```python
from build123d import *

# Parameters (mm, degrees)
BOSS_EXTRUDE1_DEPTH     = 60.96
SKETCH4_R               = 12.065
CUT_EXTRUDE3_DEPTH      = 3.81
CUT_EXTRUDE4_DEPTH      = 1
CUT_EXTRUDE4_DEPTH_BACK = 102.872142857
SKETCH7_R               = 3.81
BOSS_EXTRUDE3_DEPTH     = 3.81
CUT_EXTRUDE7_DEPTH      = 3.81
SKETCH11_R              = 12.065
CUT_EXTRUDE8_DEPTH      = 114.3


with BuildPart() as part:
    # Sketch1 → Boss-Extrude1 (new body)
    with BuildSketch(Plane.XY):
        with BuildLine():
            Line((40.776071429, -15.784285714), (40.776071429, 14.695714286))
            ThreePointArc((40.776071429, 14.695714286), (38.819326582, 21.468636013), (33.552060607, 26.154490072))
            Line((33.552060607, 26.154490072), (-40.503928571, 26.154490072))
            ThreePointArc((-40.503928571, 26.154490072), (-42.006230477, 20.457549787), (-40.776071429, 14.695714286))
            Line((-40.776071429, 14.695714286), (-40.776071429, -15.784285714))
            Line((-40.776071429, -15.784285714), (-50.936071429, -15.784285714))
            Line((-50.936071429, -15.784285714), (-50.936071429, 39.587714286))
            ThreePointArc((-50.936071429, 39.587714286), (-48.041649354, 41.212124157), (-44.960126074, 42.445250611))
            ThreePointArc((-44.960126074, 42.445250611), (-42.948064089, 46.137564922), (-42.251938956, 50.284490072))
            Line((-42.251938956, 50.284490072), (-29.309810678, 50.284490072))
            Line((-29.309810678, 50.284490072), (29.309810678, 50.284490072))
            Line((29.309810678, 50.284490072), (42.251938956, 50.284490072))
            Line((42.251938956, 50.284490072), (42.251938956, 48.042823233))
            ThreePointArc((42.251938956, 48.042823233), (45.101391865, 42.282225017), (50.936071429, 39.587714286))
            Line((50.936071429, 39.587714286), (50.936071429, -15.784285714))
            Line((50.936071429, -15.784285714), (40.776071429, -15.784285714))
        make_face()
    extrude(amount=BOSS_EXTRUDE1_DEPTH)

    # Sketch4 → Cut-Extrude3 (cut)
    with BuildSketch(Plane(origin=(0, 46.474490072, 0), x_dir=(1, 0, 0), z_dir=(0, 1, 0))):
        with Locations((0, -30.48)):
            Circle(SKETCH4_R)
    extrude(amount=-CUT_EXTRUDE3_DEPTH, mode=Mode.SUBTRACT)

    # Sketch6 → Cut-Extrude4 (cut, two sides)
    with BuildSketch(Plane(origin=(50.936071429, 0, 0), x_dir=(0, 0, -1), z_dir=(1, 0, 0))) as cut_extrude4_sk:
        with BuildLine():
            Line((-48.26, 3.773714286), (-48.26, -15.784285714))
            Line((-48.26, -15.784285714), (-12.7, -15.784285714))
            Line((-12.7, -15.784285714), (-12.7, 3.773714286))
            ThreePointArc((-12.7, 3.773714286), (-30.48, 15.984554981), (-48.26, 3.773714286))
        make_face()
    extrude(amount=CUT_EXTRUDE4_DEPTH, mode=Mode.SUBTRACT)
    extrude(cut_extrude4_sk.sketch, amount=-CUT_EXTRUDE4_DEPTH_BACK, mode=Mode.SUBTRACT)

    # Sketch7 → Boss-Extrude3 (add)
    with BuildSketch(Plane(origin=(0, 50.284490072, 0), x_dir=(1, 0, 0), z_dir=(0, 1, 0))):
        with BuildLine():
            Line((-12.20867372, -12.182150361), (-12.20867372, 0))
            Line((-12.20867372, 0), (-42.251938956, 0))
            Line((-42.251938956, 0), (-42.251938956, -60.96))
            Line((-42.251938956, -60.96), (-12.20867372, -60.96))
            Line((-12.20867372, -60.96), (-12.20867372, -48.777849639))
            Line((-12.20867372, -48.777849639), (-18.390263021, -48.777849639))
            ThreePointArc((-18.390263021, -48.777849639), (-20.904734735, -47.736321353), (-21.946263021, -45.221849639))
            Line((-21.946263021, -45.221849639), (-21.946263021, -15.738150361))
            ThreePointArc((-21.946263021, -15.738150361), (-20.904734735, -13.223678647), (-18.390263021, -12.182150361))
            Line((-18.390263021, -12.182150361), (-12.20867372, -12.182150361))
        make_face()
        with Locations((-34.250938956, -52.832)):
            Circle(SKETCH7_R, mode=Mode.SUBTRACT)
        with Locations((-34.250938956, -8.128)):
            Circle(SKETCH7_R, mode=Mode.SUBTRACT)
        with BuildLine():
            Line((42.251938956, 0), (12.20867372, 0))
            Line((12.20867372, 0), (12.20867372, -12.182150361))
            Line((12.20867372, -12.182150361), (18.390263021, -12.182150361))
            ThreePointArc((18.390263021, -12.182150361), (20.904734735, -13.223678647), (21.946263021, -15.738150361))
            Line((21.946263021, -15.738150361), (21.946263021, -45.221849639))
            ThreePointArc((21.946263021, -45.221849639), (20.904734735, -47.736321353), (18.390263021, -48.777849639))
            Line((18.390263021, -48.777849639), (12.20867372, -48.777849639))
            Line((12.20867372, -48.777849639), (12.20867372, -60.96))
            Line((12.20867372, -60.96), (42.251938956, -60.96))
            Line((42.251938956, -60.96), (42.251938956, 0))
        make_face()
        with Locations((34.250938956, -52.832)):
            Circle(SKETCH7_R, mode=Mode.SUBTRACT)
        with Locations((34.250938956, -8.128)):
            Circle(SKETCH7_R, mode=Mode.SUBTRACT)
    extrude(amount=BOSS_EXTRUDE3_DEPTH)

    # Sketch8 → Cut-Extrude7 (cut)
    with BuildSketch(Plane(origin=(0, 50.284490072, 0), x_dir=(1, 0, 0), z_dir=(0, 1, 0))):
        Polygon((-12.20867372, -12.182150361), (-18.390263021, -12.182150361), (-18.390263021, -48.777849639), (-12.20867372, -48.777849639), (12.20867372, -48.777849639), (18.390263021, -48.777849639), (18.390263021, -12.182150361), (12.20867372, -12.182150361), align=None)
        with BuildLine():
            Line((-18.390263021, -12.182150361), (-18.390263021, -48.777849639))
            ThreePointArc((-18.390263021, -48.777849639), (-20.904734735, -47.736321353), (-21.946263021, -45.221849639))
            Line((-21.946263021, -45.221849639), (-21.946263021, -15.738150361))
            ThreePointArc((-21.946263021, -15.738150361), (-20.904734735, -13.223678647), (-18.390263021, -12.182150361))
        make_face()
        with BuildLine():
            Line((18.390263021, -12.182150361), (18.390263021, -48.777849639))
            ThreePointArc((18.390263021, -48.777849639), (20.904734735, -47.736321353), (21.946263021, -45.221849639))
            Line((21.946263021, -45.221849639), (21.946263021, -15.738150361))
            ThreePointArc((21.946263021, -15.738150361), (20.904734735, -13.223678647), (18.390263021, -12.182150361))
        make_face()
    extrude(amount=-CUT_EXTRUDE7_DEPTH, mode=Mode.SUBTRACT)

    # Sketch11 → Cut-Extrude8 (cut)
    with BuildSketch(Plane(origin=(0, 0, 0), x_dir=(1, 0, 0), z_dir=(0, 1, 0))):
        with Locations((0, -30.48)):
            Circle(SKETCH11_R)
    extrude(amount=CUT_EXTRUDE8_DEPTH, mode=Mode.SUBTRACT)


solid = part.part
```
Verification items for the finished model (mm, model axes). A direction names the side the tool comes from. Round coordinates to 2 decimals unless told otherwise and drop trailing zeros. Order: outer loops, then holes, each group sorted by start corner. A loop starts at its lowest first (then second) coordinate and runs counter-clockwise, first axis right, second up.
1) Tool access check on faces 1 (the flat face through (40.776, -1, 6)), 2 (the flat face through (42.252, 51, 30)), 3 (the flat face through (-46, -6, 48.26)), 4 (the flat face through (0, 50.284, 55)), 5 (the cylindrical face through (-30.731, 52.163, 9.587)). Record the directions out of +Z, -Z, +X, -X, +Y, -Y that give a thin tool (end or side, any length) a straight path to the whole face; none if there is none.
Geometry says:
face 1: +Z, -Z, -Y
face 2: +Z, -Z, +X, +Y
face 3: +X, -X, -Y
face 4: +Z, -Z, +Y
face 5: +Y
2) Cross-section at D-D, the plane x = 15. Record the cut outline in (y, z), plus the area to 3 significant figures.
Geometry says:
outline: (26.15, 0) - (54.09, 0) - (54.09, 12.18) - (46.47, 12.18) - (46.47, 48.78) - (54.09, 48.78) - (54.09, 60.96) - (26.15, 60.96) - close
area: 1,420 mm2
3) Cross-section at A-A, the plane x = 0. Record the cut outline in (y, z) (1 decimal), plus the area to 3 significant figures.
Geometry says:
outline: (26.2, 0) - (50.3, 0) - (50.3, 12.2) - (46.5, 12.2) - (46.5, 18.4) - (26.2, 18.4) - close; (26.2, 42.5) - (46.5, 42.5) - (46.5, 48.8) - (50.3, 48.8) - (50.3, 61) - (26.2, 61) - close
area: 841 mm2
4) Cross-section at C-C, the plane y = 13. Record the cut outline in (x, z).
Geometry says:
outline: (-50.94, 0) - (-40.78, 0) - (-40.78, 20.24) - (-50.94, 20.24) - close; (-50.94, 40.72) - (-40.78, 40.72) - (-40.78, 60.96) - (-50.94, 60.96) - close; (40.78, 0) - (50.94, 0) - (50.94, 20.24) - (40.78, 20.24) - close; (40.78, 40.72) - (50.94, 40.72) - (50.94, 60.96) - (40.78, 60.96) - close
5) Material ranges on line 1 (Z direction, x = 12.5, y = 47); line 2 (X direction, y = -8, z = 7.5); line 3 (X direction, y = 39, z = 30.48) (3 decimals), recorded low to high.
Geometry says:
line 1: z = 0 to 12.18, 48.78 to 60.96
line 2: x = -50.94 to -40.78, 40.78 to 50.94
line 3: x = -50.936 to -12.065, 12.065 to 50.936
6) Depth check by flat-ended pin: pin 1 (7 mm diameter, centred on x = -34.25, z = 8.13, fed in from -Y); pin 2 (1 mm diameter, centred on x = 12.5, z = 30, fed in from +Y); pin 3 (2.5 mm diameter, centred on y = 51, z = 27, fed in from -X). Enter the tip coordinate at first touch or a pass-through.
Geometry says:
pin 1: stops at y = 26.15
pin 2: stops at y = 46.47
pin 3: stops at x = -42.26
7) Cross-section at B-B, the plane z = 28. Record the cut outline in (x, y), plus the area to 3 significant figures.
Geometry says:
outline: (-50.94, 15.82) - (-41.25, 15.82) arc R12.7 cw to (-40.5, 26.15) - (-11.81, 26.15) - (-11.81, 46.47) - (-21.95, 46.47) - (-21.95, 54.09) - (-42.25, 54.09) - (-42.25, 50.28) arc R12.7 cw to (-44.96, 42.45) arc R25.4 ccw to (-50.94, 39.59) - close; (11.81, 26.15) - (33.55, 26.15) arc R12.7 cw to (40.73, 15.82) - (50.94, 15.82) - (50.94, 39.59) arc R9.65 cw to (42.25, 48.04) - (42.25, 54.09) - (21.95, 54.09) - (21.95, 46.47) - (11.81, 46.47) - close
area: 2,050 mm2
8) Draft check along Z on faces 6 (the flat face through (-34, 50.284, 8)), 7 (the flat face through (-40.776, 0, 54)). Enter one of: +Z half, -Z half, draft (parallel to the pull), parting line (faces both ways), or undercut.
Geometry says:
face 6: undercut
face 7: draft
